from build123d import *


with BuildPart() as part:
    # Sketch1 → Revolve1 (revolve)
    with BuildSketch(Plane.XY, mode=Mode.PRIVATE) as revolve1_sk:
        with BuildLine():
            Line((-23.185394109, 10), (-25.25, 10))
            Line((-25.25, 10), (-25.25, 35))
            Line((-25.25, 35), (-14.25, 35))
            Line((-14.25, 35), (-14.25, 38))
            Line((-14.25, 38), (-5, 38))
            Line((-5, 38), (-5, 24.75))
            ThreePointArc((-5, 24.75), (-15.905808224, 19.610399403), (-23.185394109, 10))
        make_face()
    revolve(revolve1_sk.sketch.rotate(Axis((0, 108.106230536, 0), (0, -1, 0)), 270), axis=Axis((0, 108.106230536, 0), (0, -1, 0)))


solid = part.part
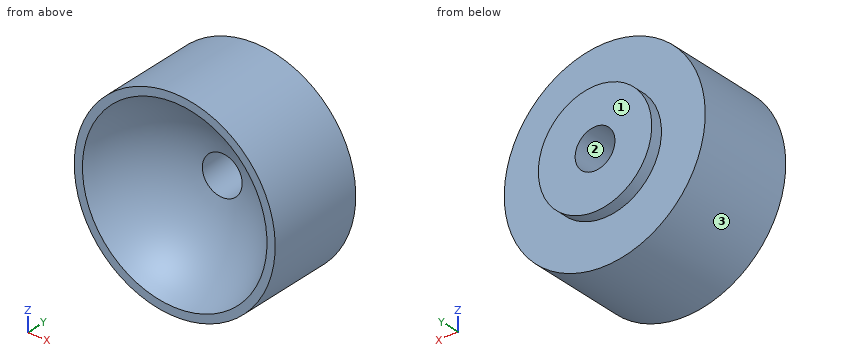
Build history of the part. All positions in model axes, mm. Face numbers are marked on the shaded views. Coordinates: 2 decimals unless noted, no trailing zeros. Write each loop counter-clockwise with the first axis right and the second up, starting at its lowest first coordinate (ties: lowest second). Pieces come first, ordered by that corner, then holes.
(1) Pin check, flat tips, straight feed: pin 1 Ø1.5 at (x, y) = (4.5, 24.5) entering from -Z; pin 2 Ø13 at (x, z) = (0, 0) entering from -Y; pin 3 Ø1 at (x, y) = (2, 24) entering from -Z. Stop position of each tip, or through.
(2) Cut at C-C on y = 30. List the corners of the cut face in (x, z).
(3) Cut at B-B on z = 0. List the corners of the cut face in (x, y).
(4) Mould opens along Z. For the marked faces 1, 2 and 3 say: pulls with the +Z half, pulls with the -Z half, needs draft (parallel to the pull), parting line crosses it, or undercut.
(5) Drill centre lines: line 1 (X direction, y = 27.5, z = 0); line 2 (Y direction, x = -19, z = 14.5); line 3 (X direction, y = 11.75, z = 17.5). Where is each one in solid material? Low to high.
(6) Cut at A-A on x = 0. List the corners of the cut face in (y, z).
(7) Cut at D-D on x = 9.5. List the corners of the cut face in (y, z), and give its area (3 significant figures).
Working result:
1. pin 1: stops at z = -24.97
1. pin 2: stops at y = 24.4
1. pin 3: stops at z = -25.21
2. outline: circle Ø50.5 at (0, 0); hole circle Ø10 at (0, 0)
3. outline: (-25.25, 10) - (-23.19, 10) arc R25.25 cw to (-5, 24.75) - (-5, 38) - (-14.25, 38) - (-14.25, 35) - (-25.25, 35) - close; (5, 24.75) arc R25.25 cw to (23.19, 10) - (25.25, 10) - (25.25, 35) - (14.25, 35) - (14.25, 38) - (5, 38) - close
4. face 1: needs draft
4. face 2: undercut
4. face 3: parting line crosses it
5. line 1: x = -25.25 to -5, 5 to 25.25
5. line 2: y = 10 to 35
5. line 3: x = -18.2 to -13.9, 13.9 to 18.2
6. outline: (10, -25.25) - (35, -25.25) - (35, -14.25) - (38, -14.25) - (38, -5) - (24.75, -5) arc R25.25 cw to (10, -23.19) - close; (10, 23.19) arc R25.25 cw to (24.75, 5) - (38, 5) - (38, 14.25) - (35, 14.25) - (35, 25.25) - (10, 25.25) - close
7. outline: (10, -23.39) - (35, -23.39) - (35, -10.62) - (38, -10.62) - (38, 10.62) - (35, 10.62) - (35, 23.39) - (10, 23.39) - (10, 21.15) arc R23.39 cw to (10, -21.15) - close
7. area: 827 mm2
